Here's the drawing with two shaded views (mm, measured from the low corner). I have some questions. Give positions to 0.01 mm unless a question says otherwise; leave off trailing zeros. Loops run counter-clockwise (first coordinate to the right, second up) from the corner with the lowest first, then second, coordinate; pieces in that order, holes last. Notation, with made-up numbers: (-17.5, 17.5) - (29.5, 17.5) arc R8 ccw to (29.5, 27.5) - close; hole circle Ø8 at (77.5, 72). An arc over 180 degrees is marked (long way). Answer as a JSON object with one key per item and string values. Group by question number.
Item 1: Suppose I cut it at A-A on x = 6. Write out the boundary of the cut face in (y, z), and give its area (3 significant figures).
Item 2: Please list where these lines run through material, in increasing order: L1, parallel to Y at x = 6, z = 6.25; L2, parallel to Y at x = 0.5, z = 2.25; L3, parallel to Y at x = 3.5, z = 6.5 (1 decimal).
Item 3: Suppose I cut it at C-C on y = 4.75. Write out the boundary of the cut face in (x, z).
Item 4: Suppose I cut it at D-D on x = 2.75. Write out the boundary of the cut face in (y, z) (1 decimal).
Item 5: Will these pins go through, and if not, where does the flat tip stop? pin 1 (1 mm diameter, centred on y = 5, z = 8, fed in from +X); pin 2 (1.1 mm diameter, centred on x = 0.5, z = 4, fed in from -Y); pin 3 (1.5 mm diameter, centred on x = 4, z = 8, fed in from -Y).
Item 6: Thinking about a two-plate mould opening in Y: for the marked faces 1, 2, 3 and 4, which applies, pulls with the +Y half, pulls with the -Y half, needs draft (parallel to the pull), parting line crosses it, or undercut?
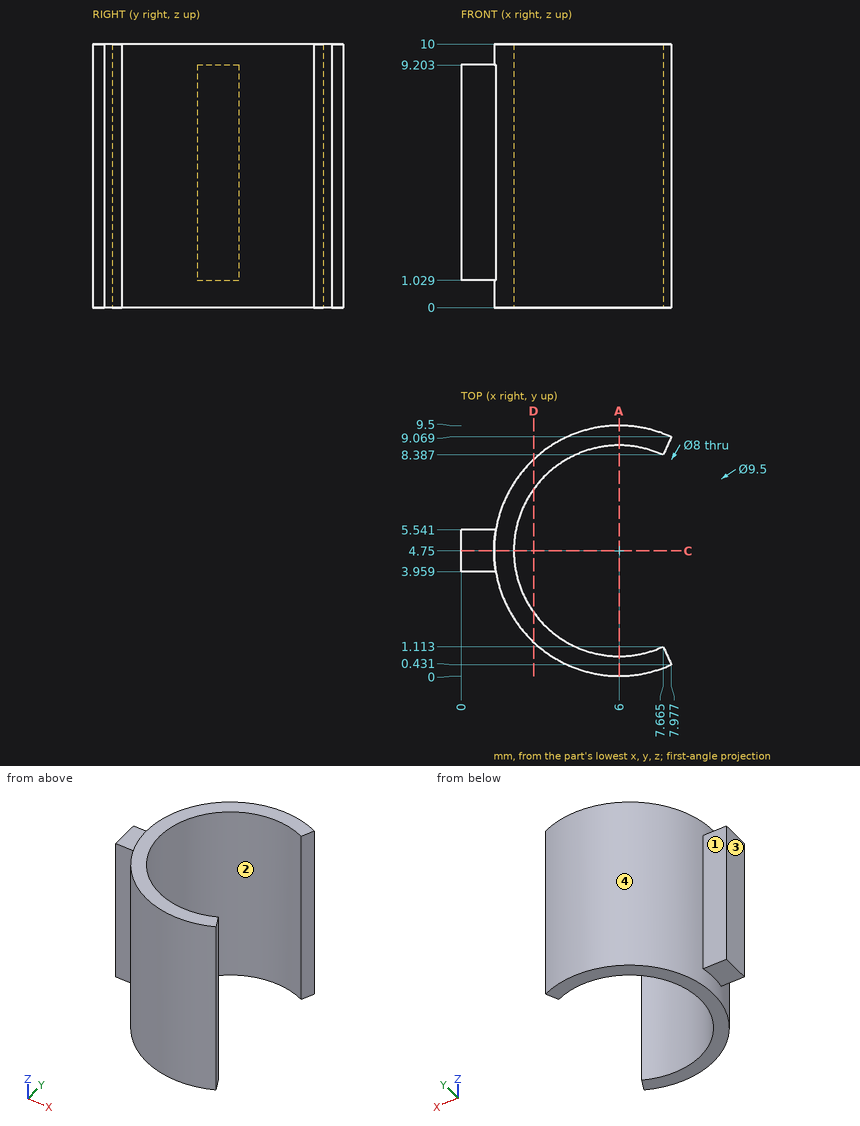
Worked out:
{
 "1": {"outline": "(0, 0) - (0.75, 0) - (0.75, 10) - (0, 10) - close; (8.75, 0) - (9.5, 0) - (9.5, 10) - (8.75, 10) - close", "area": "15.0 mm2"},
 "2": {"L1": "y = 0 to 0.75, 8.75 to 9.5", "L2": "y = 3.96 to 5.54", "L3": "y = 0.7 to 1.6, 7.9 to 8.8"},
 "3": {"outline": "(0, 1.03) - (1.25, 1.03) - (1.25, 0) - (2, 0) - (2, 10) - (1.25, 10) - (1.25, 9.2) - (0, 9.2) - close"},
 "4": {"outline": "(1.3, 0) - (2.4, 0) - (2.4, 10) - (1.3, 10) - close; (7.1, 0) - (8.2, 0) - (8.2, 10) - (7.1, 10) - close"},
 "5": {"pin 1": "stops at x = 2.07", "pin 2": "stops at y = 3.96", "pin 3": "stops at y = 0.17"},
 "6": {"face 1": "pulls with the +Y half", "face 2": "undercut", "face 3": "needs draft", "face 4": "parting line crosses it"}
}
